For this review, take the finished solid that the model builds, in its own axes (mm). Face numbers are marked on the shaded views. A direction names the side the tool comes from. Give positions to 0.01 mm unless a question says otherwise; leave off trailing zeros. Write each loop counter-clockwise with the first axis right and the second up, starting at its lowest first coordinate (ties: lowest second). Pieces come first, ordered by that corner, then holes. Notation, with made-up numbers: (38.25, -39) -> (45.25, -39) arc R17 cw to (45.25, -24) -> close; hole circle Ø3 at (74, -13.5). An arc over 180 degrees is marked (long way). Answer as CSV lines item,"result".
Autodesk Inventor part; units mm, degrees
ref_plane "YZ Plane" through (0, 0, 0) normal (1, 0, 0) x (0, 1, 0)
ref_plane "XZ Plane" through (0, 0, 0) normal (0, 1, 0) x (-1, 0, 0)
ref_plane "XY Plane" through (0, 0, 0) normal (0, 0, 1) x (1, 0, 0)
sketch "Skizze1" plane through (0, 0, 0) normal (0, 1, 0) x (-1, 0, 0)
  line L0 (-8, -8) -> (8, -8)
  line L1 (8, -8) -> (8, 8)
  line L2 (8, 8) -> (-8, 8)
  line L3 (-8, 8) -> (-8, -8)
  line L4 (-8, -8) -> (8, 8) construction
  line L5 (8, -8) -> (-8, 8) construction
  circle A0 centre (0, 0) radius 3
  line L6 (4.75, -4.75) -> (-4.75, -4.75) construction
  line L7 (-4.75, -4.75) -> (-4.75, 4.75) construction
  line L8 (-4.75, 4.75) -> (4.75, 4.75) construction
  line L9 (4.75, 4.75) -> (4.75, -4.75) construction
  line L10 (4.75, -4.75) -> (-4.75, 4.75) construction
  line L11 (-4.75, -4.75) -> (4.75, 4.75) construction
  circle A1 centre (-4.75, 4.75) radius 0.9
  circle A2 centre (-4.75, -4.75) radius 0.9
  circle A3 centre (4.75, -4.75) radius 0.9
  circle A4 centre (4.75, 4.75) radius 0.9
  dimension "d0" = 16
  dimension "d1" = 16
  dimension "d21" = 6
  dimension "d22" = 9.5
  dimension "d23" = 9.5
  dimension "d24" = 1.8
  dimension "d25" = 1.8
  dimension "d26" = 1.8
  dimension "d27" = 1.8
extrude "Extrusion1" add sketch "Skizze1" along normal blind 1
sketch "Skizze2" plane through (0, 1, 0) normal (0, 1, 0) x (1, 0, 0)
  line L0 (-8, 8) -> (-8, -8)
  line L1 (-8, -8) -> (8, -8)
  line L2 (8, -8) -> (8, 8)
  line L3 (8, 8) -> (-8, 8)
  line L4 (0, -5.1384) -> (-4.45, -2.5692)
  line L5 (-4.45, -2.5692) -> (-4.45, 2.5692)
  line L6 (-4.45, 2.5692) -> (0, 5.1384)
  line L7 (0, 5.1384) -> (4.45, 2.5692)
  line L8 (4.45, 2.5692) -> (4.45, -2.5692)
  line L9 (4.45, -2.5692) -> (0, -5.1384)
  line L10 (-8, 8) -> (-8, -8)
  line L11 (8, 8) -> (-8, 8)
  line L12 (8, -8) -> (8, 8)
  line L13 (-8, -8) -> (8, -8)
  circle A0 centre (0, 0) radius 3
  circle A1 centre (4.75, -4.75) radius 0.9
  circle A2 centre (4.75, 4.75) radius 0.9
  circle A3 centre (-4.75, 4.75) radius 0.9
  circle A4 centre (-4.75, -4.75) radius 0.9
  point P0 (8, 5.7735)
  point P1 (8, -5.7735)
  point P2 (-8, -5.7735)
  point P3 (-8, 5.7735)
  point P4 (4.1436, -8)
  point P5 (-4.1436, -8)
  point P6 (4.1436, 8)
  point P7 (-4.1436, 8)
  point P8 (-5.0758, 3.9111)
  point P9 (-3.8605, 4.6127)
  point P10 (3.8605, 4.6127)
  point P11 (5.0758, 3.9111)
  point P12 (5.0758, -3.9111)
  point P13 (3.8605, -4.6127)
  point P14 (-3.8605, -4.6127)
  point P15 (-5.0758, -3.9111)
  dimension "d6" = 8.9
extrude "Extrusion2" add sketch "Skizze2" along normal blind 9 contours L3 L2 L1 L0 | A1 | A2 | A3 | A4
fillet "Rundung2" radius 1 16 edges at (0, 5.5, 5.1384) (-4.45, 5.5, 2.5692) (-4.45, 5.5, -2.5692) (0, 5.5, -5.1384) (4.45, 5.5, -2.5692) (4.45, 5.5, 2.5692) (8, 5, -8) (-8, 5, -8) (-8, 5, 8) (8, 5, 8) (-2.225, 10, -3.8538) (-4.45, 10, 0) (-2.225, 10, 3.8538) (2.225, 10, 3.8538) (4.45, 10, 0) (2.225, 10, -3.8538)
sketch "Skizze3" plane through (0, 10, 0) normal (0, 1, 0) x (1, 0, 0)
  arc A0 (7, -8) -> (8, -7) centre (7, -7) ccw
  line L0 (8, -7) -> (8, 7)
  arc A1 (8, 7) -> (7, 8) centre (7, 7) ccw
  line L1 (7, 8) -> (-7, 8)
  arc A2 (-7, 8) -> (-8, 7) centre (-7, 7) ccw
  line L2 (-8, 7) -> (-8, -7)
  arc A3 (-8, -7) -> (-7, -8) centre (-7, -7) ccw
  line L3 (-7, -8) -> (7, -8)
  line L4 (-8, -5.6869) -> (8, -5.6869)
  line L5 (8, -5.6869) -> (8, -13.6869)
  line L6 (6, -15.6869) -> (-6, -15.6869)
  line L7 (-8, -13.6869) -> (-8, -5.6869)
  circle A4 centre (-4.925, -12.0977) radius 1.4
  circle A5 centre (2.836, -12.0977) radius 1.4
  arc A6 (-8, -13.6869) -> (-6, -15.6869) centre (-6, -13.6869) ccw
  arc A7 (6, -15.6869) -> (8, -13.6869) centre (6, -13.6869) ccw
  point P0 (0, 0)
  point P1 (8, -15.6869)
  point P2 (8, -7)
  dimension "d10" = 10
  dimension "d11" = 2.8
  dimension "d12" = 2.8
  dimension "d13" = 2
extrude "Extrusion3" add sketch "Skizze3" against normal blind 3 contours A0 L5 A7 L6 A6 L7 A3 L3
sketch "Skizze4" plane through (0, 0, 0) normal (0, -1, 0) x (1, 0, 0)
  line L0 (12.8, 30) -> (12.8, 10)
  line L1 (12.8, 30) -> (6.8, 30)
  line L2 (6.8, 10) -> (6.8, 30)
  line L3 (12.8, 10) -> (6.8, 10)
  line L4 (6.7, 30.1) -> (12.9, 30.1)
  line L5 (12.9, 30.1) -> (12.9, 9.9)
  line L6 (12.9, 9.9) -> (6.7, 9.9)
  line L7 (6.7, 9.9) -> (6.7, 30.1)
  point P0 (0, 0)
  dimension "d16" = 0.1
extrude "Extrusion4" cut sketch "Skizze4" against normal through all contours L0 L3 L2 L1 | L4 L5 L6 L7
sketch "Skizze5" plane through (0, 0, 0) normal (0, -1, 0) x (1, 0, 0)
  line L0 (-4.75, -4.75) -> (4.75, -4.75)
  line L1 (4.75, -4.75) -> (4.75, 4.75)
  line L2 (4.75, 4.75) -> (-4.75, 4.75)
  line L3 (-4.75, 4.75) -> (-4.75, -4.75)
  line L4 (-4.75, -4.75) -> (4.75, 4.75) construction
  line L5 (4.75, -4.75) -> (-4.75, 4.75) construction
  point P0 (0, 0)
  dimension "d19" = 9.5
  dimension "d20" = 9.5
hole "Bohrung1" at (4.75, 0, 4.75) at (-4.75, 0, 4.75) at (4.75, 0, -4.75) at (-4.75, 0, -4.75) direction (0, 1, 0) diameter 2 depth 8 tip angle 150
properties part number "30_Laser_to_M12Adapter_9,5mm"
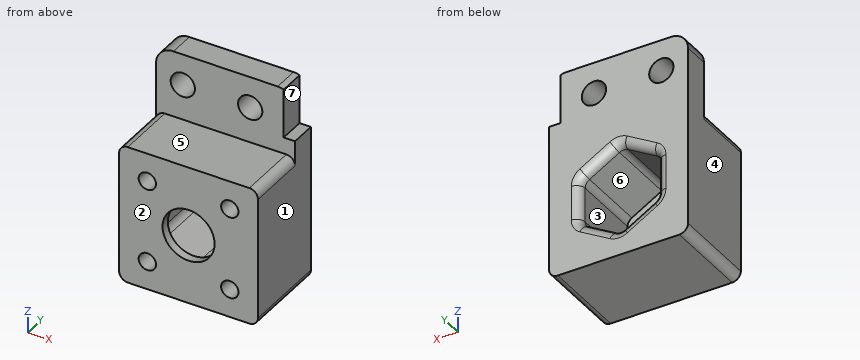
Q1. To check wall thickness, follow probe 1 along Z at (x, y) = (-4.75, 4.75); probe 2 along X at (y, z) = (2.75, 2); probe 3 along Z at (x, y) = (-5.5, 1.25). State the ranges of each line that lie inside material, in increasing order. Write a range as [from, to].
Answer block:
probe 1,"z = [-8, -5.75], [-3.75, 3.75], [5.75, 8]"
probe 2,"x = [-8, -4.45], [4.45, 8]"
probe 3,"z = [-8, -5.41], [-4.09, 4.09], [5.41, 8]"
Q2. Add section C-C (z = 0). Write out the cut boundary in (x, y), plus the area to 3 significant figures.
Answer block:
outline,"(-8, 0) -> (-3, 0) -> (-3, 1) -> (-4.45, 1) -> (-4.45, 9) arc R1 ccw to (-5.45, 10) -> (-8, 10) -> close; (3, 0) -> (8, 0) -> (8, 10) -> (5.45, 10) arc R1 ccw to (4.45, 9) -> (4.45, 1) -> (3, 1) -> close"
area,"73.5 mm2"
Q3. For the marked faces 5, 6 and 7, list the 3-axis set-ups (+Z, -Z, +X, -X, +Y, -Y) from which the entire face can be reached by the end or side of a thin tool; tool diameter is ignored.
Answer block:
face 5,"+Z, +X, -X, -Y"
face 6,"+Y"
face 7,"+Z, +X, +Y, -Y"
Q4. Draft analysis for pull direction X (two halves, no side actions). For the marked faces 1, 2, 3 and 4, state which applies: released by +X, released by -X, zero draft, split by the parting line, or undercut.
Answer block:
face 1,"released by +X"
face 2,"zero draft"
face 3,"undercut"
face 4,"released by -X"
Q5. Add section D-D (y = 9.75). Write out the cut boundary in (x, z) (3 decimals).
Answer block:
outline,"(-8, -7) arc R1 ccw to (-7, -8) -> (7, -8) arc R1 ccw to (8, -7) -> (8, 9.9) -> (6.7, 9.9) -> (6.7, 15.56) arc R2 ccw to (6, 15.687) -> (-6, 15.687) arc R2 ccw to (-8, 13.687) -> close; hole circle Ø2.8 at (-4.925, 12.098); hole (-4.789, -1.992) arc R1.339 ccw to (-4.119, -3.151) -> (-0.669, -5.143) arc R1.339 ccw to (0.669, -5.143) -> (4.119, -3.151) arc R1.339 ccw to (4.789, -1.992) -> (4.789, 1.992) arc R1.339 ccw to (4.119, 3.151) -> (0.669, 5.143) arc R1.339 ccw to (-0.669, 5.143) -> (-4.119, 3.151) arc R1.339 ccw to (-4.789, 1.992) -> close; hole circle Ø2.8 at (2.836, 12.098)"
Q6. Add section A-A (y = 4.5). Write out the cut boundary in (x, z).
Answer block:
outline,"(-8, -7) arc R1 ccw to (-7, -8) -> (7, -8) arc R1 ccw to (8, -7) -> (8, 7) arc R1 ccw to (7, 8) -> (-7, 8) arc R1 ccw to (-8, 7) -> close; hole circle Ø2 at (-4.75, -4.75); hole circle Ø2 at (-4.75, 4.75); hole (-4.45, -1.99) arc R1 ccw to (-3.95, -2.86) -> (-0.5, -4.85) arc R1 ccw to (0.5, -4.85) -> (3.95, -2.86) arc R1 ccw to (4.45, -1.99) -> (4.45, 1.99) arc R1 ccw to (3.95, 2.86) -> (0.5, 4.85) arc R1 ccw to (-0.5, 4.85) -> (-3.95, 2.86) arc R1 ccw to (-4.45, 1.99) -> close; hole circle Ø2 at (4.75, -4.75); hole circle Ø2 at (4.75, 4.75)"
Q7. Add section B-B (x = 0). Write out the cut boundary in (y, z).
Answer block:
outline,"(0, -8) -> (10, -8) -> (10, -5.98) arc R1 ccw to (9, -4.98) -> (1, -4.98) -> (1, -3) -> (0, -3) -> close; (0, 3) -> (1, 3) -> (1, 4.98) -> (9, 4.98) arc R1 ccw to (10, 5.98) -> (10, 15.69) -> (7, 15.69) -> (7, 8) -> (0, 8) -> close"
Q8. Clearance check with flat-ended pins moving along their axes: pin 1 (2.5 mm diameter, centred on x = -3.5, z = 9.5, fed in from -Y); pin 2 (1.5 mm diameter, centred on y = 8, z = 11.5, fed in from +X); pin 3 (0.6 mm diameter, centred on x = 7.5, y = 8, fed in from +Z); pin 4 (2.5 mm diameter, centred on x = 1.5, z = 0, fed in from +Y). State where each tip first meets the part, or that it passes through.
Answer block:
pin 1,"stops at y = 7"
pin 2,"stops at x = 6.7"
pin 3,"stops at z = 9.9"
pin 4,"passes through"
